Check sheet for the modelled part. Datum: model origin and axes. Units: mm. Face numbers are marked on the shaded views. A direction names the side the tool comes from. Round coordinates to 2 decimals unless told otherwise and drop trailing zeros. Write each loop counter-clockwise with the first axis right and the second up, starting at its lowest first coordinate (ties: lowest second). Pieces come first, ordered by that corner, then holes.
Item 1: Cross-section at A-A on y = 15. Enter the section's corners in (x, z).
Item 2: Release check for a two-part mould opening along X. For the marked faces 3, 4, 5 and 6 record: +X half, -X half, draft (parallel to the pull), parting line (faces both ways), or undercut.
Item 3: Cross-section at D-D on z = 15.5. Enter the section's corners in (x, y).
Item 4: Go/stop test with flat-tipped pins: pin 1 Ø12 at (x, y) = (26.5, 15.5) entering from -Z; pin 2 Ø14 at (x, y) = (60, 15) entering from +Z; pin 3 Ø4 at (y, z) = (51, 17) entering from +X. Record where each tip stops, or that it passes through.
Item 5: Cross-section at B-B on x = 30. Enter the section's corners in (y, z).
Item 6: Cross-section at C-C on y = 25. Enter the section's corners in (x, z), plus the area to 3 significant figures.
Item 7: Tool access check on the marked faces 1 and 2. Record the directions out of +Z, -Z, +X, -X, +Y, -Y that give a thin tool (end or side, any length) a straight path to the whole face; none if there is none.
Item 8: Material ranges on line 1 (Y direction, x = 30, z = 6.5); line 2 (X direction, y = 16.5, z = 6.5); line 3 (Z direction, x = 16, y = 96), recorded low to high.
from build123d import *

# Parameters (mm, degrees)
F0_W     = 75
F0_H     = 100
F1_DEPTH = 12
F4_DEPTH = 100
F6_D     = 12
F6_DEPTH = 12


with BuildPart() as f1:
    # F0 (on Top) → F1 (new body)
    with BuildSketch(Plane.XY):
        with Locations((37.5, 50)):
            Rectangle(F0_W, F0_H)
    extrude(amount=F1_DEPTH)

    # F3 (on face) → F4 (join)
    with BuildSketch(Plane.XZ):
        Polygon((0, 20), (0, 12), (16, 12), align=None)
    extrude(amount=-F4_DEPTH)

    # F6
    with Locations(Plane.XY.offset(12)):
        with Locations((30, 15), (60, 15), (60, 85), (30, 85)):
            Hole(F6_D / 2, depth=F6_DEPTH)


solid = f1.part
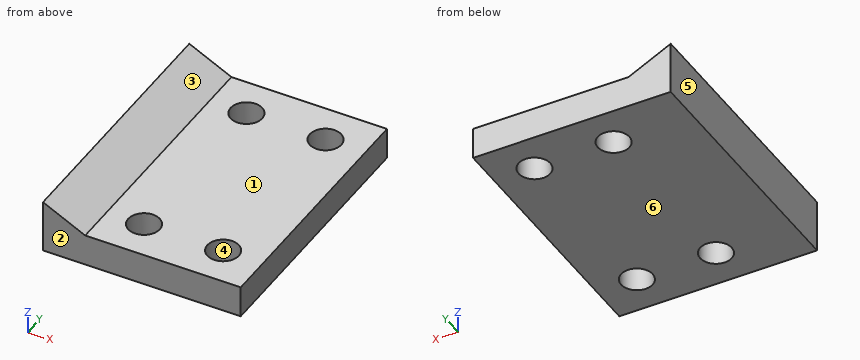
Response values:
1. outline: (0, 0) - (24, 0) - (24, 12) - (16, 12) - (0, 20) - close; (36, 0) - (54, 0) - (54, 12) - (36, 12) - close; (66, 0) - (75, 0) - (75, 12) - (66, 12) - close
2. face 3: +X half
2. face 4: undercut
2. face 5: -X half
2. face 6: draft
3. outline: (0, 0) - (9, 0) - (9, 100) - (0, 100) - close
4. pin 1: stops at z = 0
4. pin 2: stops at z = 12
4. pin 3: stops at x = 10
5. outline: (0, 0) - (9, 0) - (9, 12) - (0, 12) - close; (21, 0) - (79, 0) - (79, 12) - (21, 12) - close; (91, 0) - (100, 0) - (100, 12) - (91, 12) - close
6. outline: (0, 0) - (75, 0) - (75, 12) - (16, 12) - (0, 20) - close
6. area: 964 mm2
7. face 1: +Z, +X, +Y, -Y
7. face 2: +Z, -Z, +X, -X, -Y
8. line 1: y = 0 to 9, 21 to 79, 91 to 100
8. line 2: x = 0 to 24.19, 35.81 to 54.19, 65.81 to 75
8. line 3: z = 0 to 12
